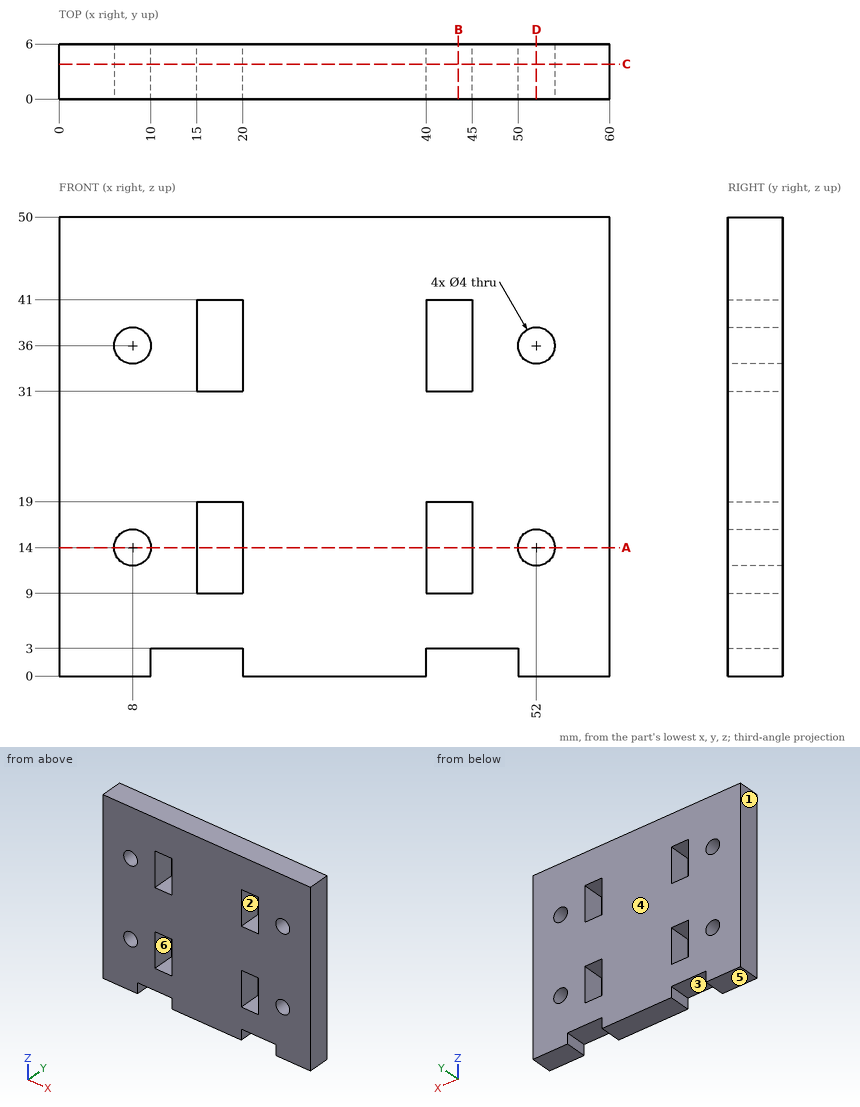
Drawing for the job (mm, zero at the part's lowest x, y, z). A direction names the side the tool comes from. Coordinates: 2 decimals unless noted, no trailing zeros. Order: outer loops, then holes, each group sorted by start corner. A loop starts at its lowest first (then second) coordinate and runs counter-clockwise, first axis right, second up. Notation, with made-up numbers: (-7, 16.5) -> (7, 16.5) arc R22 ccw to (7, 27.5) -> close; hole circle Ø11 at (3, 72). An arc over 180 degrees is marked (long way). Return JSON: item names as keys, results as strings.
Item 1: Mould opens along Z. For the marked faces 4, 5 and 6 say: pulls with the +Z half, pulls with the -Z half, needs draft (parallel to the pull), parting line crosses it, or undercut.
Model answer:
{"face 4": "needs draft", "face 5": "pulls with the -Z half", "face 6": "undercut"}
Item 2: Slice it at D-D (x = 52). Write the cut outline in (y, z).
Model answer:
{"outline": "(0, 0) -> (6, 0) -> (6, 12) -> (0, 12) -> close; (0, 16) -> (6, 16) -> (6, 34) -> (0, 34) -> close; (0, 38) -> (6, 38) -> (6, 50) -> (0, 50) -> close"}
Item 3: 3-axis set-ups, long thin cutter, end or side, ignore diameter. For the marked faces 1, 2 and 3: which of +Z, -Z, +X, -X, +Y, -Y reach the whole face in a straight line?
Model answer:
{"face 1": "+Z, -Z, -X, +Y, -Y", "face 2": "+Y, -Y", "face 3": "-Z, +Y, -Y"}
Item 4: Wall check: line 1 along X through (y, z) = (1.45, 14); line 2 along Z through (x, y) = (44, 5.35); line 3 along X through (y, z) = (1, 39.5). Give the ranges that are in metal, low to high. Write a range as from..to.
Model answer:
{"line 1": "x = 0..6, 10..15, 20..40, 45..50, 54..60", "line 2": "z = 3..9, 19..31, 41..50", "line 3": "x = 0..15, 20..40, 45..60"}
Item 5: Pin check, flat tip, straight feed: P1, Ø1.8, axis at x = 44.5, y = 2.5, coming from the -Z side. Stop position of the tip, or through.
Model answer:
{"P1": "stops at z = 3"}
Item 6: Slice it at A-A (z = 14). Write the cut outline in (x, y), then the cut area to 3 significant figures.
Model answer:
{"outline": "(0, 0) -> (6, 0) -> (6, 6) -> (0, 6) -> close; (10, 0) -> (15, 0) -> (15, 6) -> (10, 6) -> close; (20, 0) -> (40, 0) -> (40, 6) -> (20, 6) -> close; (45, 0) -> (50, 0) -> (50, 6) -> (45, 6) -> close; (54, 0) -> (60, 0) -> (60, 6) -> (54, 6) -> close", "area": "252 mm²"}
Item 7: Slice it at C-C (y = 3.8). Count the separate pieces of the cut face and the enclosed holes in it, then the cut area to 3 significant figures.
Model answer:
{"separate pieces": "1", "enclosed holes": "8", "area": "2,690 mm²"}
Item 8: Slice it at B-B (x = 43.5). Write the cut outline in (y, z).
Model answer:
{"outline": "(0, 3) -> (6, 3) -> (6, 9) -> (0, 9) -> close; (0, 19) -> (6, 19) -> (6, 31) -> (0, 31) -> close; (0, 41) -> (6, 41) -> (6, 50) -> (0, 50) -> close"}
